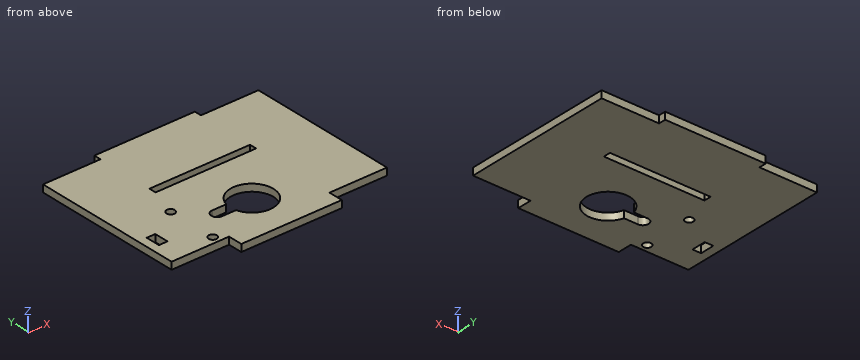
from build123d import *

# Parameters (mm, degrees)
SKETCH1_R           = 1.425
SKETCH1_W           = 3
SKETCH1_H           = 5
SKETCH1_W_2         = 35
SKETCH1_H_2         = 2.5
BOSS_EXTRUDE1_DEPTH = 2.5


with BuildPart() as part:
    # Sketch1 → Boss-Extrude1 (new body)
    with BuildSketch(Plane.XY):
        Polygon((17.5, 30), (-17.5, 30), (-17.5, 27.5), (-37.5, 27.5), (-37.5, -25), (-17.5, -25), (-17.5, -30), (17.5, -30), (17.5, -25), (37.5, -25), (37.5, 27.5), (17.5, 27.5), align=None)
        with Locations((-20.93, -5.22)):
            Circle(SKETCH1_R, mode=Mode.SUBTRACT)
        with Locations(Location((-20.93, -22.38, 0), (0, 0, 180))):
            Circle(SKETCH1_R, mode=Mode.SUBTRACT)
        with BuildLine():
            Line((-12.09, -11.8), (-7.228416147, -11.8))
            ThreePointArc((-7.228416147, -11.8), (7.5, -13.8), (-7.228416147, -15.8))
            Line((-7.228416147, -15.8), (-12.09, -15.8))
            ThreePointArc((-12.09, -15.8), (-14.09, -13.8), (-12.09, -11.8))
        make_face(mode=Mode.SUBTRACT)
        with Locations((-33, -13.8)):
            Rectangle(SKETCH1_W, SKETCH1_H, mode=Mode.SUBTRACT)
        with Locations((0, 6.25)):
            Rectangle(SKETCH1_W_2, SKETCH1_H_2, mode=Mode.SUBTRACT)
    extrude(amount=BOSS_EXTRUDE1_DEPTH)


solid = part.part
Read the model definition and answer for the solid it produces. Units are mm, in the model's axes. Coordinates: 2 decimals unless noted, no trailing zeros. Loops run counter-clockwise (first coordinate to the right, second up) from the corner with the lowest first, then second, coordinate; pieces in that order, holes last. Notation, with made-up numbers: (80.25, 62) -> (139.25, 62) arc R30 ccw to (139.25, 92) -> close; hole circle Ø3 at (-39, 3). An arc over 180 degrees is marked (long way). Answer in a Markdown table with one row per item.
Item 1: A cutting plane is placed at C-C on y = -13.8. Determine the outline of the cut face in (x, z).
Returned:
| item | result |
|---|---|
| outline | (-37.5, 0) -> (-34.5, 0) -> (-34.5, 2.5) -> (-37.5, 2.5) -> close; (-31.5, 0) -> (-14.09, 0) -> (-14.09, 2.5) -> (-31.5, 2.5) -> close; (7.5, 0) -> (37.5, 0) -> (37.5, 2.5) -> (7.5, 2.5) -> close |
Item 2: Each of these flat-tipped pins is pushed along its axis until it touches: P1, Ø1.2, axis at y = -27.5, z = 1.5, coming from the +X side; P2, Ø1.2, axis at x = 25, z = 1, coming from the +Y side. Where does it stop, or does it pass through?
Returned:
| item | result |
|---|---|
| P1 | stops at x = 17.5 |
| P2 | stops at y = 27.5 |
Item 3: A cutting plane is placed at B-B on x = 14. Determine the outline of the cut face in (y, z).
Returned:
| item | result |
|---|---|
| outline | (-30, 0) -> (5, 0) -> (5, 2.5) -> (-30, 2.5) -> close; (7.5, 0) -> (30, 0) -> (30, 2.5) -> (7.5, 2.5) -> close |
Item 4: Straight lines are drawn through the part: line 1 along Y through (x, z) = (-20.93, 1.75) (3 decimals); line 2 along Y through (x, z) = (-10, 0.3); line 3 along Y through (x, z) = (-32, 0.5). For each, find the intervals that lie inside material, in ascending order. Write a range as [from, to].
Returned:
| item | result |
|---|---|
| line 1 | y = [-25, -23.805], [-20.955, -6.645], [-3.795, 27.5] |
| line 2 | y = [-30, -15.8], [-11.8, 5], [7.5, 30] |
| line 3 | y = [-25, -16.3], [-11.3, 27.5] |
Item 5: A cutting plane is placed at D-D on x = -20.93. Determine the outline of the cut face in (y, z) (3 decimals).
Returned:
| item | result |
|---|---|
| outline | (-25, 0) -> (-23.805, 0) -> (-23.805, 2.5) -> (-25, 2.5) -> close; (-20.955, 0) -> (-6.645, 0) -> (-6.645, 2.5) -> (-20.955, 2.5) -> close; (-3.795, 0) -> (27.5, 0) -> (27.5, 2.5) -> (-3.795, 2.5) -> close |
Item 6: A cutting plane is placed at A-A on y = -5.22. Determine the outline of the cut face in (x, z) (3 decimals).
Returned:
| item | result |
|---|---|
| outline | (-37.5, 0) -> (-22.355, 0) -> (-22.355, 2.5) -> (-37.5, 2.5) -> close; (-19.505, 0) -> (37.5, 0) -> (37.5, 2.5) -> (-19.505, 2.5) -> close |
